```python
from build123d import *

# Parameters (mm, degrees)
SKETCH1_W           = 38.1
SKETCH1_H           = 393.7
BOSS_EXTRUDE1_DEPTH = 88.9
SKETCH3_R           = 3.175
CUT_EXTRUDE2_DEPTH  = 337.964070937
SKETCH2_R           = 3.175
CUT_EXTRUDE3_DEPTH  = 365.806065952


with BuildPart() as part:
    # Sketch1 → Boss-Extrude1 (new body)
    with BuildSketch(Plane(origin=(0, 0, 0), x_dir=(1, 0, 0), z_dir=(0, 1, 0))):
        with Locations((-125.830263158, 125.934703947)):
            Rectangle(SKETCH1_W, SKETCH1_H)
    extrude(amount=BOSS_EXTRUDE1_DEPTH)

    # Sketch3 → Cut-Extrude2 (cut, through all)
    with BuildSketch(Plane.ZY.offset(144.880263158)):
        with Locations((-84.532703947, 44.45)):
            Circle(SKETCH3_R)
        with Locations((-144.984703947, 44.45)):
            Circle(SKETCH3_R)
    extrude(amount=-CUT_EXTRUDE2_DEPTH, mode=Mode.SUBTRACT)

    # Sketch2 → Cut-Extrude3 (cut, through all)
    with BuildSketch(Plane(origin=(0, 0, 0), x_dir=(-1, 0, 0), z_dir=(0, -1, 0))):
        with Locations(Location((125.830263158, -26.465296053, 0), (0, 0, 90))):
            Circle(SKETCH2_R)
    extrude(amount=-CUT_EXTRUDE3_DEPTH, mode=Mode.SUBTRACT)


solid = part.part
```
Read the model definition and answer for the solid it produces. Units are mm, in the model's axes. Give positions to 0.01 mm unless a question says otherwise; leave off trailing zeros. Put each result on its own line as item: value. Start each with the question number.
1. For a pull along Y with two mould halves and no side action, classify faces 1 (the flat face through (-126, 44, -322.785)), 2 (the cylindrical face through (-126.1, 46.6, -86.87)), 3 (the flat face through (-126, 88.9, -129)) as released by +Y, released by -Y, zero draft, split by the parting line, or undercut.
2. Consider line 1 along Z through (x, y) = (-132, 44); line 2 along Z through (x, y) = (-116, 45); line 3 along Z through (x, y) = (-128, 44). Determine where each line is inside the solid, lowest interval first.
3. This flat-tipped pin is pushed along its axis until it touches: pin 1 Ø6 at (x, z) = (-132, -244.5) entering from -Y. Where does it stop, or does it pass through?
Final values:
1. face 1: zero draft
1. face 2: undercut
1. face 3: released by +Y
2. line 1: z = -322.78 to -148.13, -141.84 to -87.68, -81.39 to 70.92
2. line 2: z = -322.78 to -148.11, -141.86 to -87.66, -81.41 to 70.92
2. line 3: z = -322.78 to -148.13, -141.84 to -87.68, -81.39 to 24.15, 28.78 to 70.92
3. pin 1: stops at y = 0
